from build123d import *

# Parameters (mm, degrees)
SKETCH_R      = 13.5
PAD_DEPTH     = 2
SKETCH001_R   = 13.5
SKETCH001_R_2 = 10.85
PAD001_DEPTH  = 1
SKETCH002_R   = 13.5
SKETCH002_R_2 = 8
PAD002_DEPTH  = 5
CHAMFER_SIZE  = 1


with BuildPart() as part:
    # Sketch → Pad (new body)
    with BuildSketch(Plane.XY):
        Circle(SKETCH_R)
    extrude(amount=PAD_DEPTH)

    # Sketch001 (on Face3 of Pad) → Pad001 (join)
    with BuildSketch(Plane.XY.offset(2)):
        Circle(SKETCH001_R)
        Circle(SKETCH001_R_2, mode=Mode.SUBTRACT)
    extrude(amount=PAD001_DEPTH)

    # Sketch002 (on Face2 of Pad001) → Pad002 (join)
    with BuildSketch(Plane(origin=(0, 0, 0), x_dir=(1, 0, 0), z_dir=(0, 0, -1))):
        Circle(SKETCH002_R)
        Circle(SKETCH002_R_2, mode=Mode.SUBTRACT)
    extrude(amount=PAD002_DEPTH)

    # Chamfer
    chamfer_edges = [part.edges().sort_by_distance(p)[0] for p in [
        (-8, 0, -5),
    ]]
    chamfer(chamfer_edges, length=CHAMFER_SIZE)


solid = part.part
Model file for the job. Use its own axes, mm. A direction names the side the tool comes from. Give positions to 0.01 mm unless a question says otherwise; leave off trailing zeros. Order: outer loops, then holes, each group sorted by start corner. A loop starts at its lowest first (then second) coordinate and runs counter-clockwise, first axis right, second up. Notation, with made-up numbers: M 20,-29 L 74,-29 A29 cw 74,-1 Z; hole C 38,-32.75 d1. An arc over 180 degrees is marked long. Write item = value, one per line.
Q1. Cut at A-A, the plane x = 0. List the corners of the cut face in (y, z), then the cut area to 3 significant figures.
Derived:
outline = M -13.5,-5 L -9,-5 L -8,-4 L -8,0 L 8,0 L 8,-4 L 9,-5 L 13.5,-5 L 13.5,3 L 10.85,3 L 10.85,2 L -10.85,2 L -10.85,3 L -13.5,3 Z
area = 113 mm2
Q2. Flat gauge pins, fed straight in: pin 1 (1 mm diameter, centred on x = -5, y = -6.5, fed in from +Z); pin 2 (1 mm diameter, centred on x = 3, z = -3, fed in from -Y). Where does each tip first touch, or does it go through?
Derived:
pin_1 = 2
pin_2 = -13.27
Q3. Cut at D-D, the plane x = -11.5. List the corners of the cut face in (y, z), then the cut area to 3 significant figures.
Derived:
outline = M -7.07,-5 L 7.07,-5 L 7.07,3 L -7.07,3 Z
area = 113 mm2
Q4. Drill centre lines: line 1 (Y direction, x = 0, z = -2.85); line 2 (Y direction, x = 0, z = 2.5). Where is each one in solid material? Low to high. Write a range as [from, to].
Derived:
line_1 = [-13.5, -8], [8, 13.5]
line_2 = [-13.5, -10.85], [10.85, 13.5]
Q5. Cut at C-C, the plane x = 10. List the corners of the cut face in (y, z), then the cut area to 3 significant figures.
Derived:
outline = M -9.07,-5 L 9.07,-5 L 9.07,3 L 4.21,3 L 4.21,2 L -4.21,2 L -4.21,3 L -9.07,3 Z
area = 137 mm2
Q6. Cut at B-B, the plane z = -1. List the corners of the cut face in (x, y), then the cut area to 3 significant figures.
Derived:
outline = C 0,0 d27; hole C 0,0 d16
area = 371 mm2
Q7. Two-plate mould, pull along X, no slides. Class faces 4 (the flat face through (0, 0, 2)), 5 (the flat face through (0, 11, 3)), 6 (the cylindrical face through (-1.73, 7.81, -1.97)), 7 (the cylindrical face through (-2.93, 13.18, -0.94)): pulls with the +X half, pulls with the -X half, needs draft (parallel to the pull), parting line crosses it, or undercut.
Derived:
face_4 = undercut
face_5 = needs draft
face_6 = undercut
face_7 = parting line crosses it
Q8. Tool access for faces 1 (the flat face through (9, 3, -5)), 2 (the flat face through (0, 0, 0)), 3 (the cylindrical face through (-8, 7.33, 2.49)): list every direction of +Z, -Z, +X, -X, +Y, -Y with a clear straight run to the whole face (end or side of a thin tool).
Derived:
face_1 = -Z, +X, -X, +Y, -Y
face_2 = -Z
face_3 = +Z
